Work out the finished part from the listing and answer in its coordinate system (mm). Face numbers are marked on the shaded views. A direction names the side the tool comes from. Give positions to 0.01 mm unless a question says otherwise; leave off trailing zeros. Loops run counter-clockwise (first coordinate to the right, second up) from the corner with the lowest first, then second, coordinate; pieces in that order, holes last. Notation, with made-up numbers: M -17.5,13 L -4.5,13 A22 ccw -4.5,42 Z; hole C 36.25,37.5 d9. An arc over 180 degrees is marked long. Write item = value, one per line. Start each with the question number.
1. Consider L1, parallel to Y at x = -9, z = 6; L2, parallel to Y at x = 0, z = -6; L3, parallel to Z at x = 7.5, y = -1. Determine where each line is inside the solid, lowest interval first. Write a range as [from, to].
2. Section D-D on y = 2 is taken. Determine the outline of the cut face in (x, z), plus the area to 3 significant figures.
3. For the marked faces 4, 5 and 6, determine the directions among +Z, -Z, +X, -X, +Y, -Y from which every point of the face is accessible in a straight line to the end or side of a thin tool.
4. Section C-C on z = -6.5 is taken. Determine the outline of the cut face in (x, y), plus the area to 3 significant figures.
5. Flat-ended cylindrical pins translate along their axes: pin 1 Ø0.7 at (y, z) = (-1.5, -6.5) entering from +X; pin 2 Ø0.5 at (y, z) = (-6, -7) entering from +X; pin 3 Ø4 at (x, y) = (-5, -3) entering from +Z; pin 4 Ø3.5 at (x, z) = (-7.64, 4.47) entering from +Y. Find the tip coordinate at first contact, or state that the pin passes through.
6. The mould has two halves that part along X. Classify the marked faces 1, 2 and 3: released by +X, released by -X, zero draft, split by the parting line, or undercut.
7. Section B-B on x = -1.25 is taken. Determine the outline of the cut face in (y, z), plus the area to 3 significant figures.
8. Section A-A on y = -3.25 is taken. Give the number of separate pieces and of enclosed holes in the cut face, plus the area to 3 significant figures.
```python
from build123d import *

# Parameters (mm, degrees)
SKETCH1_W           = 20.7772
SKETCH1_H           = 15.8496
SKETCH1_R           = 1.5494
BOSS_EXTRUDE2_DEPTH = 3.2385
SKETCH2_W           = 20.4978
SKETCH2_H           = 2.54
BOSS_EXTRUDE3_DEPTH = 2.4384
SKETCH3_W           = 0.6223
SKETCH3_H           = 0.6223
BOSS_EXTRUDE4_DEPTH = 5.7404


with BuildPart() as part:
    # Sketch1 → Boss-Extrude2 (new body)
    with BuildSketch(Plane(origin=(0, 0, 0), x_dir=(1, 0, 0), z_dir=(0, 1, 0))):
        with Locations((0, 0.7239)):
            Rectangle(SKETCH1_W, SKETCH1_H)
        with Locations((7.64032, -4.46786)):
            Circle(SKETCH1_R, mode=Mode.SUBTRACT)
        with Locations((-7.64032, -4.46786)):
            Circle(SKETCH1_R, mode=Mode.SUBTRACT)
    extrude(amount=BOSS_EXTRUDE2_DEPTH)

    # Sketch2 → Boss-Extrude3 (add)
    with BuildSketch(Plane(origin=(0, 0, 0), x_dir=(1, 0, 0), z_dir=(0, 1, 0))):
        with Locations((0, 7.0485)):
            Rectangle(SKETCH2_W, SKETCH2_H)
    extrude(amount=-BOSS_EXTRUDE3_DEPTH)

    # Sketch3 → Boss-Extrude4 (add)
    with BuildSketch(Plane.XZ.offset(2.4384)):
        with Locations((-6.29285, -7.0485)):
            Rectangle(SKETCH3_W, SKETCH3_H)
        with Locations((-8.83285, -7.0485)):
            Rectangle(SKETCH3_W, SKETCH3_H)
        with Locations((-3.75285, -7.0485)):
            Rectangle(SKETCH3_W, SKETCH3_H)
        with Locations((-1.21285, -7.0485)):
            Rectangle(SKETCH3_W, SKETCH3_H)
        with Locations((1.32715, -7.0485)):
            Rectangle(SKETCH3_W, SKETCH3_H)
        with Locations((3.86715, -7.0485)):
            Rectangle(SKETCH3_W, SKETCH3_H)
        with Locations((6.40715, -7.0485)):
            Rectangle(SKETCH3_W, SKETCH3_H)
        with Locations((8.94715, -7.0485)):
            Rectangle(SKETCH3_W, SKETCH3_H)
    extrude(amount=BOSS_EXTRUDE4_DEPTH)


solid = part.part
```
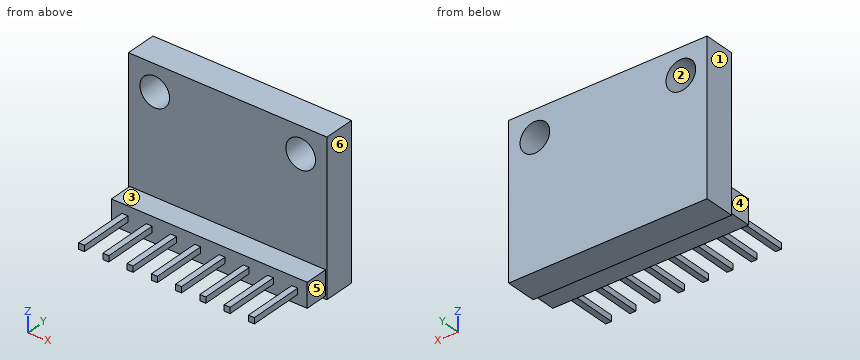
Verdict:
q1.L1 = [0, 3.24]
q1.L2 = [-2.44, 3.24]
q1.L3 = [-8.32, -5.78]
q2.outline = M -10.39,-8.65 L 10.39,-8.65 L 10.39,7.2 L -10.39,7.2 Z; hole C -7.64,4.47 d3.1; hole C 7.64,4.47 d3.1
q2.area = 314 mm2
q3.face_4 = +Z, -Z, -X, -Y
q3.face_5 = +Z, -Z, +X, -Y
q3.face_6 = +Z, -Z, +X, +Y, -Y
q4.outline = M -10.39,0 L -10.25,0 L -10.25,-2.44 L 10.25,-2.44 L 10.25,0 L 10.39,0 L 10.39,3.24 L -10.39,3.24 Z
q4.area = 117 mm2
q5.pin_1 = 10.25
q5.pin_2 = 9.26
q5.pin_3 = -5.78
q5.pin_4 = 3.24
q6.face_1 = released by -X
q6.face_2 = undercut
q6.face_3 = zero draft
q7.outline = M -8.18,-7.36 L -2.44,-7.36 L -2.44,-8.32 L 0,-8.32 L 0,-8.65 L 3.24,-8.65 L 3.24,7.2 L 0,7.2 L 0,-5.78 L -2.44,-5.78 L -2.44,-6.74 L -8.18,-6.74 Z
q7.area = 61.1 mm2
q8.separate_pieces = 8
q8.enclosed_holes = 0
q8.area = 3.10 mm2
